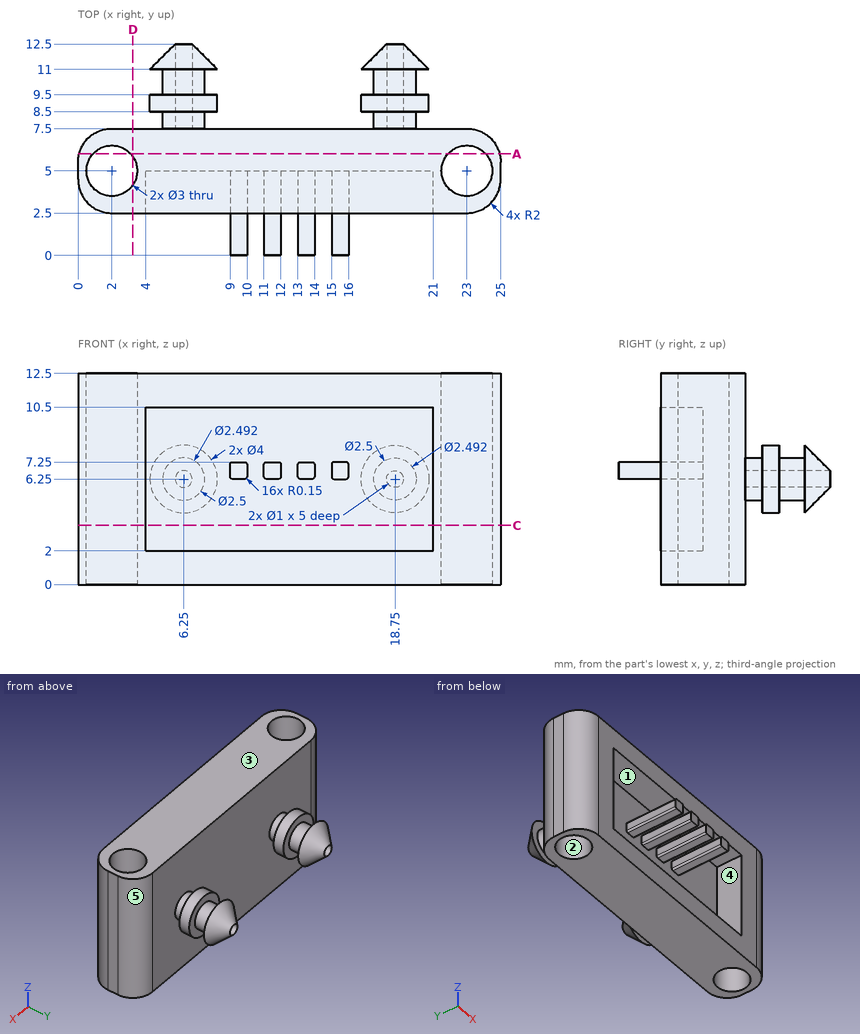
Design review of the part shown in the three views and the two pictorial views. Dimensions are in mm from the part's minimum x, y and z. A direction names the side the tool comes from. Round coordinates to 2 decimals unless told otherwise and drop trailing zeros. Write each loop counter-clockwise with the first axis right and the second up, starting at its lowest first coordinate (ties: lowest second). Pieces come first, ordered by that corner, then holes. Notation, with made-up numbers: (38, -2) -> (48, -2) arc R36 cw to (48, 37) -> close; hole circle Ø3 at (16.25, 86.5). An arc over 180 degrees is marked (long way). Use one line per item in the form item = value.
1) Take a section at D-D, the plane x = 3.25. Write out the cut boundary in (y, z).
Found:
outline = (2.5, 0) -> (4.17, 0) -> (4.17, 12.5) -> (2.5, 12.5) -> close; (5.83, 0) -> (7.5, 0) -> (7.5, 12.5) -> (5.83, 12.5) -> close
2) Mouldability with a two-part tool opening along Z and no side actions: class the marked faces 3, 4 and 5 as +Z half, -Z half, draft (parallel to the pull), parting line (faces both ways), or undercut.
Found:
face_3 = +Z half
face_4 = undercut
face_5 = draft
3) Take a section at A-A, the plane y = 6. Write out the cut boundary in (x, z), and give its area (3 significant figures).
Found:
outline = (0.06, 0) -> (0.88, 0) -> (0.88, 12.5) -> (0.06, 12.5) -> close; (3.12, 0) -> (21.88, 0) -> (21.88, 12.5) -> (3.12, 12.5) -> close; (24.12, 0) -> (24.94, 0) -> (24.94, 12.5) -> (24.12, 12.5) -> close
area = 255 mm2
4) Take a section at C-C, the plane z = 3.5. Write out the cut boundary in (x, y).
Found:
outline = (0, 4.5) arc R2 ccw to (2, 2.5) -> (4, 2.5) -> (4, 5) -> (21, 5) -> (21, 2.5) -> (23, 2.5) arc R2 ccw to (25, 4.5) -> (25, 5.5) arc R2 ccw to (23, 7.5) -> (2, 7.5) arc R2 ccw to (0, 5.5) -> close; hole circle Ø3 at (2, 5); hole circle Ø3 at (23, 5)
5) Tool access review of the marked faces 1 and 2: name each direction out of +Z, -Z, +X, -X, +Y, -Y from which nothing blocks a thin tool from reaching the whole face with its end or side.
Found:
face_1 = -Y
face_2 = +Z, -Z
6) Clearance check with flat-ended pins moving along their axes: pin 1 (0.8 mm diameter, centred on x = 9.5, y = 1.5, fed in from -Z); pin 2 (0.6 mm diameter, centred on y = 2.5, z = 7, fed in from -X) (1 decimal); pin 3 (4 mm diameter, centred on x = 4.5, z = 6.5, fed in from -Y); pin 4 (5 mm diameter, centred on x = 18, z = 8.5, fed in from +Y). State where each tip first meets the part, or that it passes through.
Found:
pin_1 = 6.25
pin_2 = 0.9
pin_3 = 2.5
pin_4 = 12.5
7) To check wall thickness, follow L1, parallel to X at y = 9.4, z = 6.25; L2, parallel to Y at x = 2, z = 10.25; L3, parallel to Y at x = 10.5, z = 8.5. State the ranges of each line that lie inside material, in increasing order. Write a range as from..to.
Found:
L1 = 4.25..5.75, 6.75..8.25, 16.75..18.25, 19.25..20.75
L2 = 2.5..3.5, 6.5..7.5
L3 = 5..7.5
